```python
from build123d import *

# Parameters (mm, degrees)
SKETCH_1_R               = 19
EXTRUDE_1_DEPTH          = 3
CUT_EXTRUDE_1_REACH      = 29.037
SKETCH_2_R               = 1.6
SKETCH_3_W               = 4
SKETCH_3_H               = 20
EXTRUDE_2_DEPTH          = 20
SKETCH_4_W               = 90
SKETCH_4_H               = 90
EXTRUDE_3_DEPTH          = 5
CUT_EXTRUDE_2_DEPTH      = 70.526973183
CUT_EXTRUDE_2_DEPTH_BACK = 70.526973183
SKETCH_5_R               = 3.3
CUT_EXTRUDE_3_DEPTH      = 70.526973183
CUT_EXTRUDE_3_DEPTH_BACK = 5
SKETCH_6_W               = 22
SKETCH_6_H               = 30


with BuildPart() as part:
    # 草图1 → 凸台-拉伸1 (new body)
    with BuildSketch(Plane(origin=(0, 0, 0), x_dir=(1, 0, 0), z_dir=(0, 1, 0))):
        with Locations(Location((0, 0, 0), (0, 0, 270))):
            Circle(SKETCH_1_R)
    extrude(amount=EXTRUDE_1_DEPTH)

    # 草图2 → 切除-拉伸1 (cut, up to next)
    with BuildSketch(Plane(origin=(0, 3, 0), x_dir=(1, 0, 0), z_dir=(0, 1, 0)), mode=Mode.PRIVATE) as cut_extrude_1_sk1:
        with Locations(Location((-5, 0, 0), (0, 0, 270))):
            Circle(SKETCH_2_R)
    cut_extrude_1_tool1 = extrude(cut_extrude_1_sk1.sketch, amount=-CUT_EXTRUDE_1_REACH, mode=Mode.PRIVATE) & part.part
    # 草图2 → 切除-拉伸1 (cut, up to next)
    with BuildSketch(Plane(origin=(0, 3, 0), x_dir=(1, 0, 0), z_dir=(0, 1, 0)), mode=Mode.PRIVATE) as cut_extrude_1_sk2:
        with Locations(Location((0, 0, 0), (0, 0, 270))):
            Circle(SKETCH_2_R)
    cut_extrude_1_tool2 = extrude(cut_extrude_1_sk2.sketch, amount=-CUT_EXTRUDE_1_REACH, mode=Mode.PRIVATE) & part.part
    # 草图2 → 切除-拉伸1 (cut, up to next)
    with BuildSketch(Plane(origin=(0, 3, 0), x_dir=(1, 0, 0), z_dir=(0, 1, 0)), mode=Mode.PRIVATE) as cut_extrude_1_sk3:
        with Locations(Location((5, 0, 0), (0, 0, 270))):
            Circle(SKETCH_2_R)
    cut_extrude_1_tool3 = extrude(cut_extrude_1_sk3.sketch, amount=-CUT_EXTRUDE_1_REACH, mode=Mode.PRIVATE) & part.part
    # 草图2 → 切除-拉伸1 (cut, up to next)
    with BuildSketch(Plane(origin=(0, 3, 0), x_dir=(1, 0, 0), z_dir=(0, 1, 0)), mode=Mode.PRIVATE) as cut_extrude_1_sk4:
        with Locations(Location((0, -5, 0), (0, 0, 270))):
            Circle(SKETCH_2_R)
    cut_extrude_1_tool4 = extrude(cut_extrude_1_sk4.sketch, amount=-CUT_EXTRUDE_1_REACH, mode=Mode.PRIVATE) & part.part
    add(cut_extrude_1_tool1.solids().sort_by_distance((-5, 3, 0))[0], mode=Mode.SUBTRACT)
    add(cut_extrude_1_tool2.solids().sort_by_distance((0, 3, 0))[0], mode=Mode.SUBTRACT)
    add(cut_extrude_1_tool3.solids().sort_by_distance((5, 3, 0))[0], mode=Mode.SUBTRACT)
    add(cut_extrude_1_tool4.solids().sort_by_distance((0, 3, 5))[0], mode=Mode.SUBTRACT)

    # 草图3 → 凸台-拉伸2 (add)
    with BuildSketch(Plane(origin=(0, 3, 0), x_dir=(1, 0, 0), z_dir=(0, 1, 0))):
        with Locations((-13, 0)):
            Rectangle(SKETCH_3_W, SKETCH_3_H)
        with Locations((13, 0)):
            Rectangle(SKETCH_3_W, SKETCH_3_H)
    extrude(amount=EXTRUDE_2_DEPTH)

    # 草图4 → 凸台-拉伸3 (add)
    with BuildSketch(Plane(origin=(0, 23, 0), x_dir=(1, 0, 0), z_dir=(0, 1, 0))):
        Rectangle(SKETCH_4_W, SKETCH_4_H)
    extrude(amount=EXTRUDE_3_DEPTH)

    # 草图5 → 切除-拉伸2 (cut, two sides: drawn at the far end of the back side and taken through both)
    with BuildSketch(Plane(origin=(0, 28, 0), x_dir=(1, 0, 0), z_dir=(0, 1, 0)).offset(-CUT_EXTRUDE_2_DEPTH_BACK)):
        with Locations(Location((-38, 38, 0), (0, 0, 270))):
            Circle(SKETCH_5_R)
        with Locations(Location((38, 38, 0), (0, 0, 270))):
            Circle(SKETCH_5_R)
        with Locations(Location((-38, -38, 0), (0, 0, 270))):
            Circle(SKETCH_5_R)
        with Locations(Location((38, -38, 0), (0, 0, 270))):
            Circle(SKETCH_5_R)
    extrude(amount=CUT_EXTRUDE_2_DEPTH + CUT_EXTRUDE_2_DEPTH_BACK, mode=Mode.SUBTRACT)

    # 草图6 → 切除-拉伸3 (cut, two sides: drawn at the far end of the back side and taken through both)
    with BuildSketch(Plane(origin=(0, 28, 0), x_dir=(1, 0, 0), z_dir=(0, 1, 0)).offset(-CUT_EXTRUDE_3_DEPTH_BACK)):
        Rectangle(SKETCH_6_W, SKETCH_6_H)
    extrude(amount=CUT_EXTRUDE_3_DEPTH + CUT_EXTRUDE_3_DEPTH_BACK, mode=Mode.SUBTRACT)


solid = part.part
```
Verification items for the finished model (mm, model axes). A direction names the side the tool comes from. Coordinates: 2 decimals unless noted, no trailing zeros. Loops run counter-clockwise (first coordinate to the right, second up) from the corner with the lowest first, then second, coordinate; pieces in that order, holes last. Notation, with made-up numbers: (80, 47.25) - (121, 47.25) arc R16 ccw to (121, 74.25) - close; hole circle Ø7 at (65.5, 84.5). An arc over 180 degrees is marked (long way). Return JSON: item names as keys, results as strings.
1. Section check D-D, the plane y = 14.25. Record the boundary of the cut face in (x, z).
Established:
{"outline": "(-15, -10) - (-11, -10) - (-11, 10) - (-15, 10) - close; (11, -10) - (15, -10) - (15, 10) - (11, 10) - close"}
2. Tool access check on faces 4 (the flat face through (13, 13, -10)), 5 (the flat face through (-15, 13, 0)), 6 (the cylindrical face through (-11.56, 1.48, -15.08)), 7 (the flat face through (-11, 15, 0)). Record the directions out of +Z, -Z, +X, -X, +Y, -Y that give a thin tool (end or side, any length) a straight path to the whole face; none if there is none.
Established:
{"face 4": "-Z, +X, -X", "face 5": "+Z, -Z, -X", "face 6": "-Y", "face 7": "+Y"}
3. Thickness scan on L1, parallel to X at y = 25.2, z = -38; L2, parallel to X at y = 2, z = 0. Record the ranges inside material, lowest first.
Established:
{"L1": "x = -45 to -41.3, -34.7 to 34.7, 41.3 to 45", "L2": "x = -19 to -6.6, -3.4 to -1.6, 1.6 to 3.4, 6.6 to 19"}
4. Section check B-B, the plane x = 38. Record the boundary of the cut face in (y, z), then the cut area to 3 significant figures.
Established:
{"outline": "(23, -45) - (28, -45) - (28, -41.3) - (23, -41.3) - close; (23, -34.7) - (28, -34.7) - (28, 34.7) - (23, 34.7) - close; (23, 41.3) - (28, 41.3) - (28, 45) - (23, 45) - close", "area": "384 mm2"}
5. Section check A-A, the plane z = -38. Record the boundary of the cut face in (x, y).
Established:
{"outline": "(-45, 23) - (-41.3, 23) - (-41.3, 28) - (-45, 28) - close; (-34.7, 23) - (34.7, 23) - (34.7, 28) - (-34.7, 28) - close; (41.3, 23) - (45, 23) - (45, 28) - (41.3, 28) - close"}
6. Mould release check, pull along Z, two halves, no side actions. Record for faces 1 (the flat face through (0, 3, -4)), 2 (the flat face through (-1, 25, -45)), 3 (the flat face through (11, 15, 0)): +Z half, -Z half, draft (parallel to the pull), parting line (faces both ways), or undercut.
Established:
{"face 1": "draft", "face 2": "-Z half", "face 3": "undercut"}
7. Go/stop test with flat-tipped pins: pin 1 (3 mm diameter, centred on x = -12, z = -1, fed in from -Y); pin 2 (7.5 mm diameter, centred on y = 13.5, z = -1, fed in from +X); pin 3 (2 mm diameter, centred on x = 14, y = 12.5, fed in from +Z); pin 4 (6 mm diameter, centred on y = 17.5, z = 2.5, fed in from -X). Record where each tip stops, or that it passes through.
Established:
{"pin 1": "stops at y = 0", "pin 2": "stops at x = 15", "pin 3": "stops at z = 10", "pin 4": "stops at x = -15"}
8. Section check C-C, the plane z = 0. Record the boundary of the cut face in (x, y), then the cut area to 3 significant figures.
Established:
{"outline": "(-45, 23) - (-15, 23) - (-15, 3) - (-19, 3) - (-19, 0) - (-6.6, 0) - (-6.6, 3) - (-11, 3) - (-11, 28) - (-45, 28) - close; (-3.4, 0) - (-1.6, 0) - (-1.6, 3) - (-3.4, 3) - close; (1.6, 0) - (3.4, 0) - (3.4, 3) - (1.6, 3) - close; (6.6, 0) - (19, 0) - (19, 3) - (15, 3) - (15, 23) - (45, 23) - (45, 28) - (11, 28) - (11, 3) - (6.6, 3) - close", "area": "585 mm2"}
